from build123d import *

# Parameters (mm, degrees)
ESQUISSE1_W             = 202
ESQUISSE1_H             = 150
BOSS_EXTRU_1_DEPTH      = 4
ESQUISSE2_W             = 4
ESQUISSE2_H             = 60
ESQUISSE2_W_2           = 60
ESQUISSE2_H_2           = 4
BOSS_EXTRU_2_DEPTH      = 4
ENL_V_MAT_EXTRU_1_DEPTH = 10
ENL_V_MAT_EXTRU_2_DEPTH = 4


with BuildPart() as part:
    # Esquisse1 → Boss.-Extru.1 (new body)
    with BuildSketch(Plane.XY):
        Rectangle(ESQUISSE1_W, ESQUISSE1_H)
    extrude(amount=BOSS_EXTRU_1_DEPTH)

    # Esquisse2 → Boss.-Extru.2 (add)
    with BuildSketch(Plane(origin=(0, 0, 0), x_dir=(-1, 0, 0), z_dir=(0, 0, -1))):
        with Locations((-103, 0)):
            Rectangle(ESQUISSE2_W, ESQUISSE2_H)
        with Locations((103, 0)):
            Rectangle(ESQUISSE2_W, ESQUISSE2_H)
        with Locations((0, -77)):
            Rectangle(ESQUISSE2_W_2, ESQUISSE2_H_2)
        with Locations((0, 77)):
            Rectangle(ESQUISSE2_W_2, ESQUISSE2_H_2)
    extrude(amount=-BOSS_EXTRU_2_DEPTH)

    # Esquisse3 → Enlèv. mat.-Extru.1 (cut)
    with BuildSketch(Plane(origin=(0, 0, 0), x_dir=(-1, 0, 0), z_dir=(0, 0, -1))):
        Polygon((42.4, 75), (45.6, 75), (45.6, 72), (46.85, 72), (46.85, 67.8), (45.6, 67.8), (45.6, 64), (42.4, 64), (42.4, 67.8), (41.15, 67.8), (41.15, 72), (42.4, 72), align=None)
        Polygon((-36.6, 75), (-33.4, 75), (-33.4, 72), (-32.15, 72), (-32.15, 67.8), (-33.4, 67.8), (-33.4, 64), (-36.6, 64), (-36.6, 67.8), (-37.85, 67.8), (-37.85, 72), (-36.6, 72), align=None)
        Polygon((-33.4, -75), (-33.4, -72), (-32.15, -72), (-32.15, -67.8), (-33.4, -67.8), (-33.4, -64), (-36.6, -64), (-36.6, -67.8), (-37.85, -67.8), (-37.85, -72), (-36.6, -72), (-36.6, -75), align=None)
        Polygon((45.6, -75), (45.6, -72), (46.85, -72), (46.85, -67.8), (45.6, -67.8), (45.6, -64), (42.4, -64), (42.4, -67.8), (41.15, -67.8), (41.15, -72), (42.4, -72), (42.4, -75), align=None)
    extrude(amount=-ENL_V_MAT_EXTRU_1_DEPTH, mode=Mode.SUBTRACT)

    # Esquisse4 → Enlèv. mat.-Extru.2 (cut)
    with BuildSketch(Plane.XY.offset(4)):
        Polygon((90, 48.4), (93, 48.4), (93, 47.15), (97.2, 47.15), (97.2, 48.4), (101, 48.4), (101, 51.6), (97.2, 51.6), (97.2, 52.85), (93, 52.85), (93, 51.6), (90, 51.6), align=None)
        Polygon((97.2, -51.6), (101, -51.6), (101, -48.4), (97.2, -48.4), (97.2, -47.15), (93, -47.15), (93, -48.4), (90, -48.4), (90, -51.6), (93, -51.6), (93, -52.85), (97.2, -52.85), align=None)
        Polygon((-90, -48.4), (-93, -48.4), (-93, -47.15), (-97.2, -47.15), (-97.2, -48.4), (-101, -48.4), (-101, -51.6), (-97.2, -51.6), (-97.2, -52.85), (-93, -52.85), (-93, -51.6), (-90, -51.6), align=None)
        Polygon((-97.2, 51.6), (-101, 51.6), (-101, 48.4), (-97.2, 48.4), (-97.2, 47.15), (-93, 47.15), (-93, 48.4), (-90, 48.4), (-90, 51.6), (-93, 51.6), (-93, 52.85), (-97.2, 52.85), align=None)
    extrude(amount=-ENL_V_MAT_EXTRU_2_DEPTH, mode=Mode.SUBTRACT)


solid = part.part
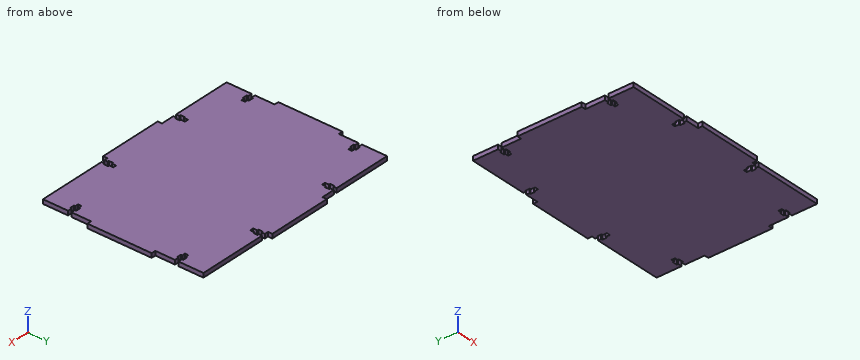
Could you check a few things on this model? Use its own coordinates, in mm. Give positions to 0.01 mm unless a question says otherwise; leave off trailing zeros. Order: outer loops, then holes, each group sorted by start corner. A loop starts at its lowest first (then second) coordinate and runs counter-clockwise, first axis right, second up. Notation, with made-up numbers: (16, 87.25) - (48, 87.25) arc R30 cw to (48, 113.25) - close; hole circle Ø10 at (19, -12). An arc over 180 degrees is marked (long way). Return JSON: item names as keys, results as strings. Group by question number.
Q1. Please list where these lines run through material, in increasing order: line 1 along Y through (x, z) = (94, 1.75); line 2 along X through (y, z) = (69.5, 2.1); line 3 along X through (y, z) = (-66, 0.2). Write a range as [from, to].
Q2. Suppose I cut it at B-B, the plane y = 40.5. Please give me the cut outline in (x, z), and give its area (3 significant figures).
Q3. Suppose I cut it at A-A, the plane x = 78. Please give me the cut outline in (y, z), and give its area (3 significant figures).
Q4. Will these pins go through, and if not, where does the flat tip stop? pin 1 Ø1.1 at (y, z) = (66.5, 2.5) entering from -X; pin 2 Ø1.2 at (x, z) = (102, 1.5) entering from +Y; pin 3 Ø1.2 at (y, z) = (77.5, 1) entering from -X.
Resolved:
{
 "1": {"line 1": "y = [-75, -52.85], [-47.15, 47.15], [52.85, 75]", "line 2": "x = [-101, -46.85], [-41.15, 32.15], [37.85, 101]", "line 3": "x = [-101, -45.6], [-42.4, 33.4], [36.6, 101]"},
 "2": {"outline": "(-101, 0) - (101, 0) - (101, 4) - (-101, 4) - close", "area": "808 mm2"},
 "3": {"outline": "(-75, 0) - (75, 0) - (75, 4) - (-75, 4) - close", "area": "600 mm2"},
 "4": {"pin 1": "stops at x = -101", "pin 2": "stops at y = 30", "pin 3": "stops at x = -30"}
}
